Answer from the drawing. Dimensions are ordinates in mm from the lowest x, y and z of the part. A direction names the side the tool comes from. Give positions to 0.01 mm unless a question says otherwise; leave off trailing zeros. Loops run counter-clockwise (first coordinate to the right, second up) from the corner with the lowest first, then second, coordinate; pieces in that order, holes last. Notation, with made-up numbers: (-5.75, 82) - (20.25, 82) arc R31 cw to (20.25, 117) - close; hole circle Ø8 at (-37.75, 67). An arc over 180 degrees is marked (long way). Write each question's results on one line, items separated by ' | '. Start each with the question number.
Q1. The part is cut by section C-C, the plane x = 19.25. Write down the section's boundary in (y, z), plus the area to 3 significant figures.
Q2. The part is cut by section B-B, the plane x = 26. Write down the section's boundary in (y, z), plus the area to 4 significant figures.
Q3. Find the intervals of material crossed by line 1 (Z direction, x = 19.25, y = 3); line 2 (Z direction, x = 38, y = 9.75); line 3 (Y direction, x = 18, z = 34), in increasing order. Write a range as from..to.
Q4. The part is cut by section A-A, the plane y = 5. Write down the section's boundary in (x, z).
Q5. The part is cut by section D-D, the plane y = 9. Write down the section's boundary in (x, z).
Q6. Given pin 1 (6 mm diameter, centred on x = 19, z = 17, fed in from +Y); pin 2 (2 mm diameter, centred on x = 32.75, z = 15, fed in from +Y); pin 3 (3 mm diameter, centred on x = 43, y = 8, fed in from -Z); pin 4 (6 mm diameter, centred on x = 32, y = 11.5, fed in from -Z), each flat-ended and moving along its own axis, determine where each tip first touches the part or whether it passes through.
Q7. For the marked faces 1 and 2, determine the directions among +Z, -Z, +X, -X, +Y, -Y from which every point of the face is accessible in a straight line to the end or side of a thin tool.
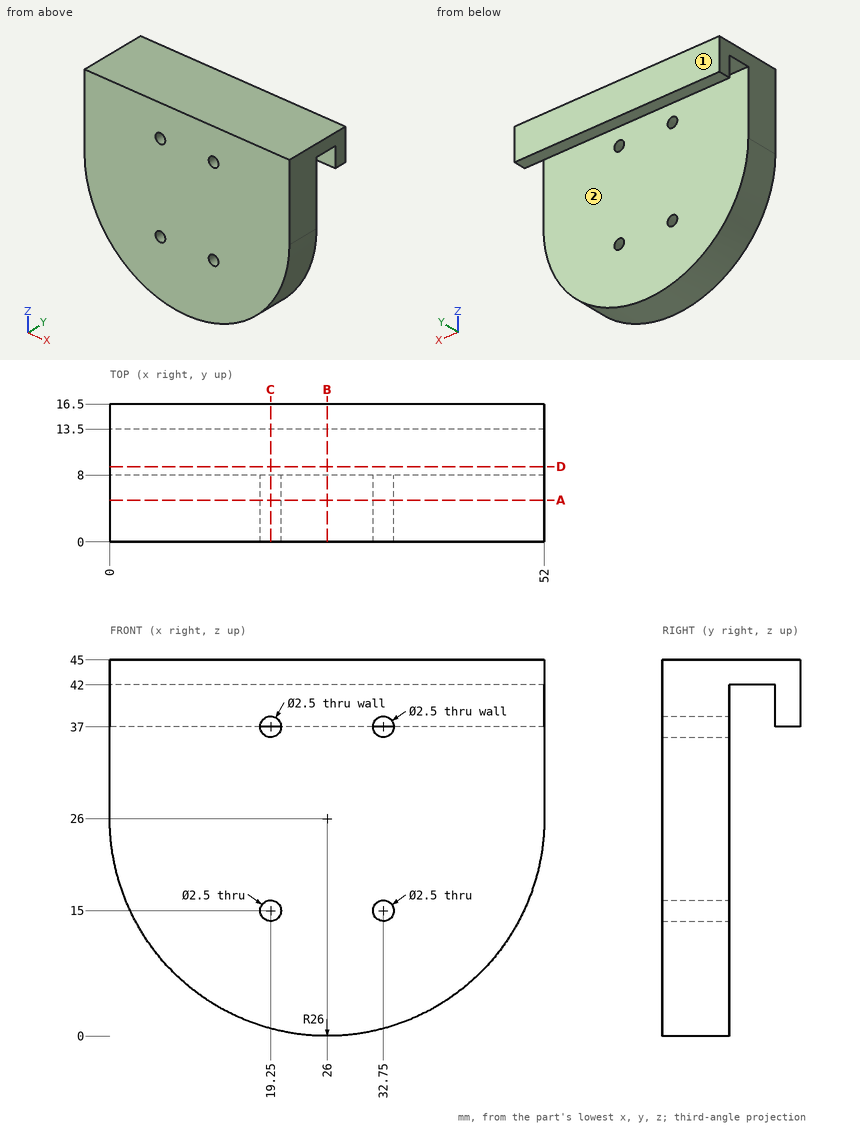
Check sheet entries:
1) outline: (0, 0.89) - (8, 0.89) - (8, 13.75) - (0, 13.75) - close; (0, 16.25) - (8, 16.25) - (8, 35.75) - (0, 35.75) - close; (0, 38.25) - (8, 38.25) - (8, 42) - (13.5, 42) - (13.5, 37) - (16.5, 37) - (16.5, 45) - (0, 45) - close | area: 353 mm^2
2) outline: (0, 0) - (8, 0) - (8, 42) - (13.5, 42) - (13.5, 37) - (16.5, 37) - (16.5, 45) - (0, 45) - close | area: 400.5 mm^2
3) line 1: z = 0.89..13.75, 16.25..35.75, 38.25..45 | line 2: z = 42..45 | line 3: y = 0..8
4) outline: (0, 26) arc R26 ccw to (52, 26) - (52, 45) - (0, 45) - close; hole circle Ø2.5 at (19.25, 15); hole circle Ø2.5 at (19.25, 37); hole circle Ø2.5 at (32.75, 15); hole circle Ø2.5 at (32.75, 37)
5) outline: (0, 42) - (52, 42) - (52, 45) - (0, 45) - close
6) pin 1: stops at y = 8 | pin 2: passes through | pin 3: stops at z = 5.13 | pin 4: stops at z = 37
7) face 1: +Z, -Z, +X, -X, +Y | face 2: -Z, +X, -X
